CAD build for the part. Positions are in the model's coordinates, mm. Give positions to 0.01 mm unless a question says otherwise; leave off trailing zeros. Order: outer loops, then holes, each group sorted by start corner. A loop starts at its lowest first (then second) coordinate and runs counter-clockwise, first axis right, second up. Notation, with made-up numbers: M -20.75,32.5 L -4.75,32.5 A10 cw -4.75,44.5 Z; hole C 27,71.5 d10. An arc over 180 degrees is marked long. Put each result on its own line as item: value. Start each with the question number.
1) Cut at B-B (z = -3.42). Write the cut outline in (x, y), and give its area (3 significant figures).
2) Drill centre lines: line 1 (X direction, y = 0.65, z = -3.42); line 2 (X direction, y = 0.35, z = -3.75). Where is each one in solid material? Low to high. Write a range as [from, to].
3) Two-plate mould, pull along Z, no slides. Class faces 1 (the face through (0, 0, 8)), 2 (the face through (-0.065, 0.02, 6.244)), 3 (the face through (-3.5, 0, 0)), 4 (the face through (0, 0, -8)): released by +Z, released by -Z, zero draft, split by the parting line, or undercut.
4) Cut at C-C (y = -0.75). Write the cut outline in (x, z), and give its area (3 significant figures).
5) Cut at A-A (x = 0). Write the cut outline in (y, z).
```python
from build123d import *

# Parameters (mm, degrees)
SKETCH1_W           = 7
SKETCH1_H           = 16
BOSS_EXTRUDE1_DEPTH = 1.45
SKETCH2_R           = 0.5
CUT_EXTRUDE1_DEPTH  = 3.9
LPATTERN1_COUNT     = 12
LPATTERN1_PITCH     = 2.54


with BuildPart() as part:
    # Sketch1 → Boss-Extrude1 (new body, symmetric)
    with BuildSketch(Plane(origin=(0, 0, 0), x_dir=(1, 0, 0), z_dir=(0, 1, 0))):
        Rectangle(SKETCH1_W, SKETCH1_H)
    extrude(amount=BOSS_EXTRUDE1_DEPTH, both=True)

    # Sketch2 → Cut-Extrude1 (cut, through all)
    with BuildSketch(Plane(origin=(0, 1.45, 0), x_dir=(1, 0, 0), z_dir=(0, 1, 0))):
        with Locations((0, 5.96)):
            Circle(SKETCH2_R)
    cut_extrude1 = extrude(amount=-CUT_EXTRUDE1_DEPTH, mode=Mode.SUBTRACT)

    # LPattern1: Cut-Extrude1 ×12
    with Locations(*[(0, 0, i * LPATTERN1_PITCH) for i in range(1, LPATTERN1_COUNT)]):
        add(cut_extrude1, mode=Mode.SUBTRACT)


solid = part.part
```
Solution:
1. outline: M -3.5,-1.45 L -0.5,-1.45 L -0.5,1.45 L -3.5,1.45 Z; M 0.5,-1.45 L 3.5,-1.45 L 3.5,1.45 L 0.5,1.45 Z
1. area: 17.4 mm²
2. line 1: [-3.5, -0.5], [0.5, 3.5]
2. line 2: [-3.5, -0.38], [0.38, 3.5]
3. face 1: released by +Z
3. face 2: undercut
3. face 3: zero draft
3. face 4: released by -Z
4. outline: M -3.5,-8 L 3.5,-8 L 3.5,8 L -3.5,8 Z; hole C 0,-5.96 d1; hole C 0,-3.42 d1; hole C 0,-0.88 d1; hole C 0,1.66 d1; hole C 0,4.2 d1; hole C 0,6.74 d1
4. area: 107 mm²
5. outline: M -1.45,-8 L 1.45,-8 L 1.45,-6.46 L -1.45,-6.46 Z; M -1.45,-5.46 L 1.45,-5.46 L 1.45,-3.92 L -1.45,-3.92 Z; M -1.45,-2.92 L 1.45,-2.92 L 1.45,-1.38 L -1.45,-1.38 Z; M -1.45,-0.38 L 1.45,-0.38 L 1.45,1.16 L -1.45,1.16 Z; M -1.45,2.16 L 1.45,2.16 L 1.45,3.7 L -1.45,3.7 Z; M -1.45,4.7 L 1.45,4.7 L 1.45,6.24 L -1.45,6.24 Z; M -1.45,7.24 L 1.45,7.24 L 1.45,8 L -1.45,8 Z
